Autodesk Fusion 360 part; units mm, degrees
sketch "Sketch1" plane through (0, 0, 0) normal (0, 0, 1) x (1, 0, 0)
  line L0 (50, 35) -> (-50, 35)
  line L1 (-50, 35) -> (-50, -35)
  line L2 (-50, -35) -> (50, -35)
  line L3 (50, -35) -> (50, 35)
  line L4 (50, 35) -> (-50, -35) construction
  line L5 (-50, 35) -> (50, -35) construction
  line L6 (-30, 35) -> (-30, 85)
  line L7 (-30, 85) -> (30, 85)
  line L8 (30, 85) -> (30, 35)
  circle A0 centre (-22, -10.5) radius 11
  circle A1 centre (22, -10.5) radius 11
  point P0 (-37.5, -26)
  point P1 (-6.5, -26)
  point P2 (-37.5, 5)
  point P3 (-6.5, 5)
  point P4 (6.5, -26)
  point P5 (37.5, -26)
  point P6 (6.5, 5)
  point P7 (37.5, 5)
  point P8 (-40, 23)
  point P9 (15, 23)
  point P10 (10, 48.9294)
  point P11 (10, 68.9294)
  point P12 (-10, 68.9294)
  point P13 (-10, 48.9294)
  point P14 (0, 35)
  point P15 (0, 60)
  dimension "d1" = 100
  dimension "d2" = 70
  dimension "d3" = 9
  dimension "d6" = 31
  dimension "d7" = 31
  dimension "d8" = 12.5
  dimension "d10" = 31
  dimension "d13" = 12.5
  dimension "d15" = 12
  dimension "d16" = 10
  dimension "d17" = 55
  dimension "d18" = 50
  dimension "d19" = 60
  dimension "d20" = 20
  dimension "d21" = 20
  dimension "d22" = 20
  dimension "d23" = 20
  dimension "d37" = 22
  dimension "d38" = 15.5
  dimension "d39" = 15.5
  dimension "d40" = 22
  dimension "d41" = 15.5
  dimension "d42" = 21.9203
  dimension "d45" = 25
extrude "Extrude1" add sketch "Sketch1" against normal blind 8 contours L0 L1 L2 L3 | L0 L6 L7 L8 | A0 | A1
hole "Hole1" at (-37.5, 5, 0) at (-37.5, -26, 0) at (-6.5, -26, 0) at (6.5, -26, 0) at (-6.5, 5, 0) at (6.5, 5, 0) at (37.5, 5, 0) at (37.5, -26, 0) at (-10, 48.9294, 0) at (-10, 68.9294, 0) at (0, 60, 0) at (10, 68.9294, 0) at (0, 35, 0) at (10, 48.9294, 0) direction (0, 0, -1) diameter 2.529 depth 40 tip angle 118
hole "Hole2" at (15, 23, 0) at (-40, 23, 0) direction (0, 0, -1) diameter 4.234 depth 20 tip angle 118
extrude "Extrude2" cut sketch "Sketch1" against normal blind 20 contours A0 | A1
equation "d38 = ( 31 / 2 ) * 1 mm"
equation "d39 = ( 31 / 2 ) * 1 mm"
equation "d41 = ( 31 / 2 ) * 1 mm"
equation "d42 = ( 31 / 2 * sqrt(2) ) * 1 mm"
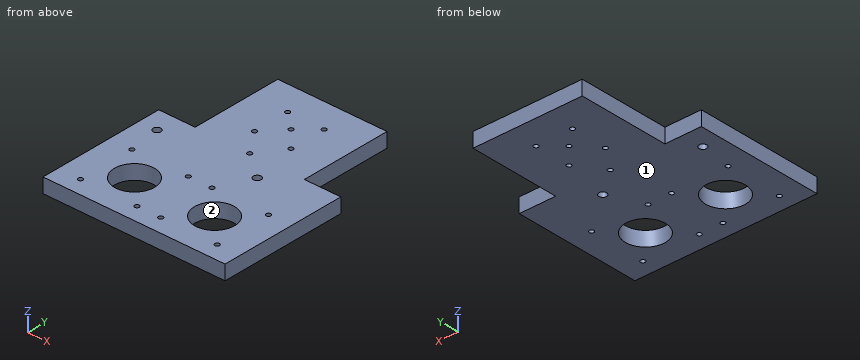
For this review, take the finished solid that the model builds, in its own axes (mm). Face numbers are marked on the shaded views. Round coordinates to 2 decimals unless told otherwise and drop trailing zeros. Write each loop counter-clockwise with the first axis right and the second up, starting at its lowest first coordinate (ties: lowest second). Pieces come first, ordered by that corner, then holes. Notation, with made-up numbers: (-35, -30) - (24, -30) arc R31 cw to (24, 8) - close; hole circle Ø5 at (-19.75, 2). An arc over 180 degrees is marked (long way). Write item = value, one per line. Start each with the question number.
1. Consider section C-C on y = 23. State the section outline as (x, z) points.
2. Draft analysis for pull direction X (two halves, no side actions). For the marked faces 1 and 2, state which applies: released by +X, released by -X, zero draft, split by the parting line, or undercut.
3. Consider section A-A on y = -26. State the section outline as (x, z) points.
4. Consider section D-D on x = 6.5. State the section outline as (y, z) points.
5. Consider section B-B on x = 22. State the section outline as (y, z) points.
6. For pin 1 Ø2.5 at (y, z) = (57.5, -4.5) entering from +X; pin 2 Ø1.5 at (x, y) = (0, 60) entering from -Z; pin 3 Ø4 at (x, z) = (-40, -2) entering from +Y; pin 4 Ø2.5 at (y, z) = (50, -3) entering from -X, all flat-tipped, find the tip position at first contact; note any pin that passes through.
7. Wall thickness on L1, parallel to Y at x = 0, z = -5.5; L2, parallel to Y at x = -10, z = -2.25; L3, parallel to X at y = 5, z = -5.5: over which ranges is each line inside the solid? List them lowest first.
Evaluation:
q1.outline = (-50, -8) - (-42.12, -8) - (-42.12, 0) - (-50, 0) - close; (-37.88, -8) - (12.88, -8) - (12.88, 0) - (-37.88, 0) - close; (17.12, -8) - (50, -8) - (50, 0) - (17.12, 0) - close
q2.face_1 = zero draft
q2.face_2 = undercut
q3.outline = (-50, -8) - (-38.76, -8) - (-38.76, 0) - (-50, 0) - close; (-36.24, -8) - (-7.76, -8) - (-7.76, 0) - (-36.24, 0) - close; (-5.24, -8) - (5.24, -8) - (5.24, 0) - (-5.24, 0) - close; (7.76, -8) - (36.24, -8) - (36.24, 0) - (7.76, 0) - close; (38.76, -8) - (50, -8) - (50, 0) - (38.76, 0) - close
q4.outline = (-35, -8) - (-27.26, -8) - (-27.26, 0) - (-35, 0) - close; (-24.74, -8) - (3.74, -8) - (3.74, 0) - (-24.74, 0) - close; (6.26, -8) - (85, -8) - (85, 0) - (6.26, 0) - close
q5.outline = (-35, -8) - (-21.5, -8) - (-21.5, 0) - (-35, 0) - close; (0.5, -8) - (85, -8) - (85, 0) - (0.5, 0) - close
q6.pin_1 = 30
q6.pin_2 = through
q6.pin_3 = 35
q6.pin_4 = -30
q7.L1 = -35 to 33.74, 36.26 to 58.74, 61.26 to 85
q7.L2 = -35 to 47.66, 50.19 to 67.66, 70.19 to 85
q7.L3 = -50 to -38.76, -36.24 to -7.76, -5.24 to 5.24, 7.76 to 36.24, 38.76 to 50
